Autodesk Inventor part; units mm, degrees
ref_plane "YZ Plane" through (0, 0, 0) normal (1, 0, 0) x (0, 1, 0)
ref_plane "XZ Plane" through (0, 0, 0) normal (0, 1, 0) x (-1, 0, 0)
ref_plane "XY Plane" through (0, 0, 0) normal (0, 0, 1) x (1, 0, 0)
sketch "草圖1" plane through (0, 0, 0) normal (1, 0, 0) x (0, 1, 0)
  line L0 (0, 0) -> (0, 65)
  line L1 (0, 65) -> (65, 0)
  line L2 (65, 0) -> (0, 0)
  line L3 (10, 55) -> (0, 55)
  line L4 (55, 10) -> (55, 0)
  line L5 (55, 10) -> (55, 55)
  line L6 (55, 55) -> (10, 55)
  dimension "d0" = 65
  dimension "d1" = 65
  dimension "d20" = 55
extrude "擠出1" add sketch "草圖1" along normal blind 20 contours L0 L3 L1 L4 L2 | L6 L5 L1
sketch "草圖2" plane through (0, 0, 0) normal (0, -1, 0) x (1, 0, 0)
  line L0 (0, 0) -> (20, 0)
  point P0 (10, 30)
  point P1 (10, 0)
  dimension "d4" = 30
hole "孔1" at (10, 0, 30) direction (0, 1, 0) diameter 4 end through all
sketch "草圖3" plane through (0, 0, 0) normal (0, 0, -1) x (-1, 0, 0)
  line L0 (0, 0) -> (-20, 0)
  point P0 (-10, 30)
  point P1 (-10, 0)
  dimension "d12" = 30
hole "孔2" at (10, 30, 0) direction (0, 0, 1) diameter 3 end through all
sketch "草圖6" plane through (0, 55, 55) normal (0, 1, 0) x (1, 0, 0)
  circle A0 centre (10, 25) radius 2
  circle A1 centre (10, 25) radius 4
  point P0 (0, 55)
  dimension "d27" = 8
extrude "擠出4" cut sketch "草圖6" against normal blind 50
sketch "草圖7" plane through (0, 0, 55) normal (0, 0, 1) x (1, 0, 0)
  circle A0 centre (10, 30) radius 1.5
  circle A1 centre (10, 30) radius 1.5
  circle A2 centre (10, 30) radius 3
  point P0 (0, 0)
  dimension "d30" = 6
extrude "擠出5" cut sketch "草圖7" against normal blind 50
sketch "草圖8" plane through (20, 0, 0) normal (1, 0, 0) x (0, 0, -1)
  line L0 (0, 0) -> (0, 55)
  line L1 (-55, 0) -> (0, 0)
  arc A0 (0, 40) -> (-40, 0) centre (0, 0) ccw
  line L2 (-55, 55) -> (-55, 0)
  line L3 (-55, 0) -> (0, 0)
  line L4 (0, 0) -> (0, 55)
  line L5 (0, 55) -> (-55, 55)
  dimension "d34" = 40
extrude "擠出6" cut sketch "草圖8" against normal through all contours A0 L1 L2 L5 L0
equation "\"d1\" = d0"
properties part number "鋁擠固定器"
Work out the finished part from the listing and answer in its coordinate system (mm). A direction names the side the tool comes from. Give positions to 0.01 mm unless a question says otherwise; leave off trailing zeros. Order: outer loops, then holes, each group sorted by start corner. A loop starts at its lowest first (then second) coordinate and runs counter-clockwise, first axis right, second up. Notation, with made-up numbers: (41, -15) -> (79, -15) arc R18 cw to (79, -11) -> close; hole circle Ø7 at (80, 75.5). An arc over 180 degrees is marked (long way). One line per item, written item: value.
Item 1: Find section B-B, the plane y = 30. Give the vertices of the cut face in (x, z), plus the area to 3 significant figures.
Answer sheet:
outline: (0, 0) -> (8.5, 0) -> (8.5, 5) -> (7, 5) -> (7, 26.46) -> (0, 26.46) -> close; (11.5, 0) -> (20, 0) -> (20, 26.46) -> (13, 26.46) -> (13, 5) -> (11.5, 5) -> close
area: 385 mm²
Item 2: A tool of negligible diameter and unlimited length cuts with its end or side. For faces 1 (the cylindrical face through (9.35, 27.07, 16.28)), 2 (the cylindrical face through (9.93, 28.5, 2.54)), 3 (the flat face through (11, 5, 28)), from which of +Z, -Z, +X, -X, +Y, -Y can it reach the whole face along a straight path? Write none if from no direction.
Answer sheet:
face 1: +Z
face 2: +Z, -Z
face 3: +Y
Item 3: Flat-ended cylindrical pins translate along their axes: P1, Ø2.5, axis at x = 8, z = 31.5, coming from the +Y side; P2, Ø1, axis at x = 5, y = 28.5, coming from the +Z side. Find the tip coordinate at first contact, or state that the pin passes through.
Answer sheet:
P1: y = 5
P2: z = 28.57
Item 4: Find section D-D, the plane z = 20. Give the vertices of the cut face in (x, y), plus the area to 3 significant figures.
Answer sheet:
outline: (0, 0) -> (20, 0) -> (20, 34.64) -> (0, 34.64) -> close; hole circle Ø6 at (10, 30)
area: 665 mm²
Item 5: Find section A-A, the plane z = 30. Give the vertices of the cut face in (x, y).
Answer sheet:
outline: (0, 0) -> (8, 0) -> (8, 5) -> (6, 5) -> (6, 26.46) -> (0, 26.46) -> close; (12, 0) -> (20, 0) -> (20, 26.46) -> (14, 26.46) -> (14, 5) -> (12, 5) -> close
Item 6: Find section C-C, the plane x = 9.5. Give the vertices of the cut face in (y, z).
Answer sheet:
outline: (0, 0) -> (28.59, 0) -> (28.59, 5) -> (27.04, 5) -> (27.04, 26.03) -> (5, 26.03) -> (5, 28.06) -> (0, 28.06) -> close; (0, 31.94) -> (5, 31.94) -> (5, 33.97) -> (21.12, 33.97) arc R40 ccw to (0, 40) -> close; (31.41, 0) -> (40, 0) arc R40 ccw to (32.96, 22.67) -> (32.96, 5) -> (31.41, 5) -> close
Item 7: Determine the mould class of faces 4 (the flat face through (0, 15, 16)), 5 (the flat face through (11.3, 28.7, 5)), 6 (the flat face through (20, 15, 16)) for opening direction X: released by +X, released by -X, zero draft, split by the parting line, or undercut.
Answer sheet:
face 4: released by -X
face 5: undercut
face 6: released by +X
Item 8: Straight lines are drawn through the part: probe 1 along X at (y, z) = (19.5, 30); probe 2 along X at (y, z) = (30, 3.3); probe 3 along Z at (x, y) = (10, 19.25). For each, find the intervals that lie inside material, in ascending order.
Answer sheet:
probe 1: 0 to 6, 14 to 20
probe 2: 0 to 8.5, 11.5 to 20
probe 3: 0 to 26, 34 to 35.06
